Check sheet for the drawn part. Datum: minimum x, y, z corner. Units: mm. Round coordinates to 2 decimals unless told otherwise and drop trailing zeros. Write each loop counter-clockwise with the first axis right and the second up, starting at its lowest first coordinate (ties: lowest second). Pieces come first, ordered by that corner, then holes. Notation, with made-up numbers: (61.5, -6.5) -> (96.5, -6.5) arc R9 cw to (96.5, 0.5) -> close; hole circle Ø11 at (60.5, 37.25). An arc over 180 degrees is marked (long way). Use a Markdown table: item, result.
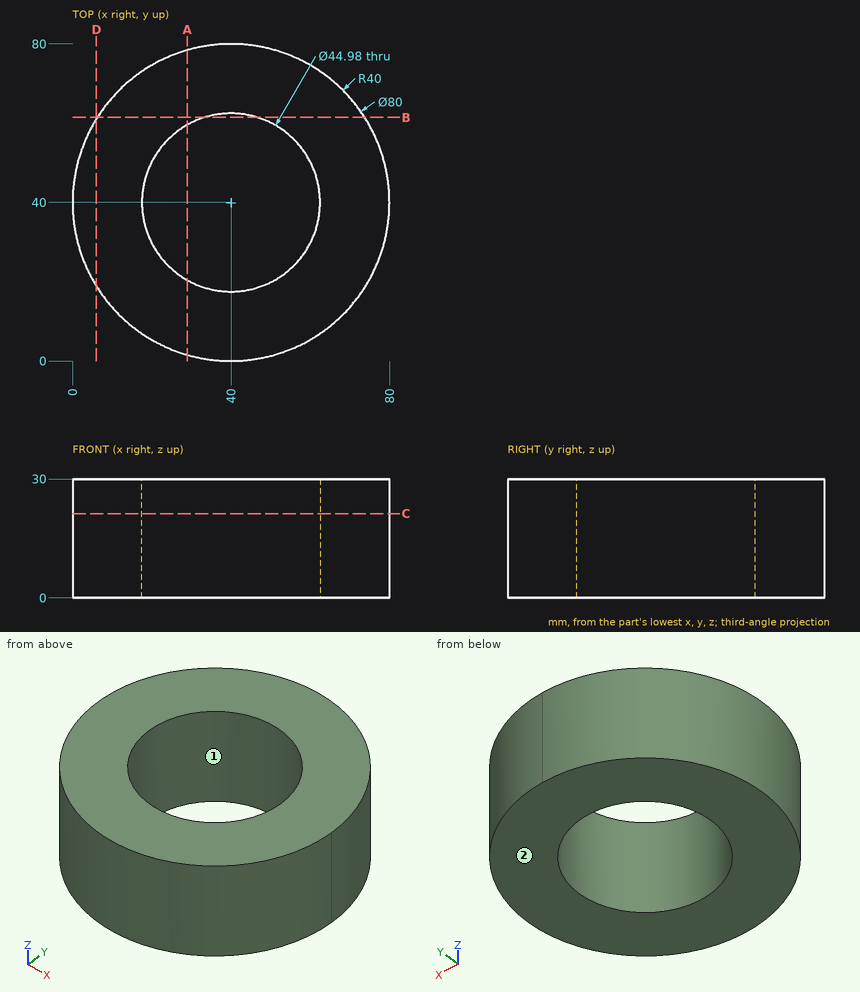
(1) Thickness scan on line 1 (X direction, y = 40, z = 11); line 2 (Y direction, x = 35, z = 16.25). Record the ranges inside material, lowest first.
A:
| item | result |
|---|---|
| line 1 | x = 0 to 17.51, 62.49 to 80 |
| line 2 | y = 0.31 to 18.07, 61.93 to 79.69 |
(2) Section check B-B on y = 61.5. Record the cut outline in (x, z).
A:
| item | result |
|---|---|
| outline | (6.27, 0) -> (33.4, 0) -> (33.4, 30) -> (6.27, 30) -> close; (46.6, 0) -> (73.73, 0) -> (73.73, 30) -> (46.6, 30) -> close |
(3) Section check D-D on x = 6. Record the cut outline in (y, z), plus the area to 3 significant figures.
A:
| item | result |
|---|---|
| outline | (18.93, 0) -> (61.07, 0) -> (61.07, 30) -> (18.93, 30) -> close |
| area | 1,260 mm2 |
(4) Section check C-C on z = 21.25. Record the cut outline in (x, y).
A:
| item | result |
|---|---|
| outline | circle Ø80 at (40, 40); hole circle Ø44.98 at (40, 40) |
(5) Release check for a two-part mould opening along Y. For the marked faces 1 and 2 record: +Y half, -Y half, draft (parallel to the pull), parting line (faces both ways), or undercut.
A:
| item | result |
|---|---|
| face 1 | undercut |
| face 2 | draft |
(6) Gauge pin test, flat ends, axial feed: pin 1 Ø1 at (y, z) = (60, 25.5) entering from +X (1 decimal); pin 2 Ø5 at (y, z) = (9.5, 22.5) entering from +X (1 decimal); pin 3 Ø2 at (y, z) = (15.5, 19) entering from +X. Record the tip position at first contact, or that the pin passes through.
A:
| item | result |
|---|---|
| pin 1 | stops at x = 74.9 |
| pin 2 | stops at x = 68.6 |
| pin 3 | stops at x = 72.37 |
(7) Section check A-A on x = 29. Record the cut outline in (y, z), plus the area to 3 significant figures.
A:
| item | result |
|---|---|
| outline | (1.54, 0) -> (20.38, 0) -> (20.38, 30) -> (1.54, 30) -> close; (59.62, 0) -> (78.46, 0) -> (78.46, 30) -> (59.62, 30) -> close |
| area | 1,130 mm2 |
